Verification items for the finished model (mm, model axes). A direction names the side the tool comes from. Round coordinates to 2 decimals unless told otherwise and drop trailing zeros. Order: outer loops, then holes, each group sorted by start corner. A loop starts at its lowest first (then second) coordinate and runs counter-clockwise, first axis right, second up. Notation, with made-up numbers: (35, 64.5) -> (52, 64.5) arc R18 ccw to (52, 74.5) -> close; hole circle Ø10 at (9, 72.25). An arc over 180 degrees is marked (long way). Put each result on its own line as item: value.
Autodesk Inventor part; units mm, degrees
ref_plane "Work Plane1" through (29, 0, 0) normal (0, -1, 0) x (1, 0, 0)
ref_plane "YZ Plane" through (0, 0, 0) normal (1, 0, 0) x (0, 1, 0)
ref_plane "XZ Plane" through (0, 0, 0) normal (0, 1, 0) x (-1, 0, 0)
sketch "Sketch1" plane through (0, 0, 0) normal (0, 0, 1) x (1, 0, 0)
  line L0 (0.4667, 0) -> (20, 0)
  line L1 (20, 0) -> (20, 4)
  line L2 (20, 4) -> (1, 4)
  line L3 (1, 4) -> (0.2331, 4)
  line L4 (0.2331, 4) -> (0, 4)
  line L5 (0, 4) -> (0, 6.5)
  line L6 (0, 6.5) -> (-5, 6.5)
  line L7 (-5, 6.5) -> (-5, 2.8868)
  line L8 (-5, 2.8868) -> (-1.2, 2.8868)
  line L9 (-1.2, 2.8868) -> (0.4667, 0)
  line L10 (-7.5, 0) -> (27.5, 0)
  line L11 (0, -0.65) -> (0, 8.45)
  line L12 (1, 4) -> (0, 4) construction
  dimension "d1" = 19
  dimension "d2" = 0.7669
  dimension "d3" = 5
  dimension "d4" = 3.8
  dimension "d5" = 60
  dimension "d6" = 8
  dimension "d7" = 8
  dimension "d8" = 5.7735
  dimension "d9" = 13
  dimension "d26" = 20
revolve "Body" add sketch "Sketch1" angle 360 about axis through (0.4667, 0, 0) along (1, 0, 0) contours L9 L11 L4 L3 L2 L1 L0 | L9 L8 L7 L6 L5 L11
sketch "Sketch2" plane through (-5, 0, 0) normal (-1, 0, 0) x (0, 0, 1)
  circle A0 centre (0, 0) radius 2.8868
  line L0 (0, -7.8) -> (0, 10.4)
  line L1 (-7.8, 0) -> (10.4, 0)
  line L2 (2.8868, 0) -> (1.4434, -2.5)
  line L3 (1.4434, -2.5) -> (-1.4434, -2.5)
  line L4 (-1.4434, -2.5) -> (-2.8868, 0)
  line L5 (-2.8868, 0) -> (-1.4434, 2.5)
  line L6 (-1.4434, 2.5) -> (1.4434, 2.5)
  line L7 (1.4434, 2.5) -> (2.8868, 0)
  point P0 (0, 0)
extrude "Slot" add sketch "Sketch2" against normal up to next contours L7 A0 | A0 L2 | L6 L0 A0 | A0 L0 L3 | L0 L6 A0 | A0 L3 L0 | L4 A0 | A0 L5
fillet "Fillet1" radius 0.8 1 edges at (-5, -6.5, 0)
thread "Thread"
chamfer "Chamfer1" distance 0.7668 distance2 0.7668 1 edges at (20, -4, 0) measured on face at (20, -0.0467, 2.2623)
ref_plane "Work Plane1" through (29, 0, 0) normal (0, -1, 0) x (1, 0, 0)
equation "\"d17\" = RR"
equation "\"d15\" = -0.5 * SPD + 0.5 * GD"
equation "\"d16\" = GUL"
equation "\"d1\" = GEL"
equation "\"d3\" = KOH"
equation "\"d4\" = INTI"
equation "\"d6\" = GD"
equation "\"d7\" = BDM"
equation "\"d8\" = 1.1547 * SW"
equation "\"d9\" = KOD"
equation "\"d26\" = NLG"
equation "\"GD\" = NND"
equation "\"NLG\" = 20"
equation "\"GEL\" = 19"
equation "\"KOD\" = 13"
equation "\"KOH\" = 5"
equation "\"INTI\" = 3.8"
equation "\"GAL\" = 0.61345 * PTC"
equation "\"GUL\" = 0.61345 * PTC"
equation "\"BDM\" = NND"
equation "\"SW\" = 5"
equation "\"RR\" = 0.8"
equation "\"SPD\" = NND - 1.2269 * PTC"
equation "\"TOA\" = 30deg"
equation "\"GD1\" = THREADDIA - 1.2269 * PTC"
equation "\"THREADDIA\" = 8"
equation "\"FAWI\" = 45deg"
equation "\"ANG\" = 120deg"
equation "\"PTC\" = 1.25"
equation "\"NND\" = 8"
equation "\"E0\" = 1.155 * SW"
properties part number "21.1202" material "Steel, Mild"
Item 1: Release check for a two-part mould opening along Y. For faces 1 (the face through (20, 0, 0)), 2 (the face through (9.482, -0.867, 3.905)), 3 (the face through (-3, 2.5, 0)) record: pulls with the +Y half, pulls with the -Y half, needs draft (parallel to the pull), parting line crosses it, or undercut.
Geometry check:
face 1: needs draft
face 2: parting line crosses it
face 3: undercut
Item 2: Sectioned sample at A-A, the plane x = 3.5. Record the boundary of the cut face in (y, z).
Geometry check:
outline: circle Ø8 at (0, 0)
Item 3: Tool access check on faces 4 (the face through (0, 3, 3)), 5 (the face through (-3.017, 1.268, 2.155)), 6 (the face through (-2.129, -5.158, 3.955)). Record the directions out of +Z, -Z, +X, -X, +Y, -Y that give a thin tool (end or side, any length) a straight path to the whole face; none if there is none.
Geometry check:
face 4: +X
face 5: -X
face 6: +X, -X
Item 4: Material ranges on line 1 along X through (y, z) = (4.75, 2); line 2 along X through (y, z) = (-4.25, 4.75); line 3 along Z through (x, y) = (3.25, 3.25), recorded low to high.
Geometry check:
line 1: -5 to 0
line 2: -4.63 to 0
line 3: -2.33 to 2.33
Item 5: Depth check by flat-ended pin: pin 1 Ø6 at (x, y) = (14.5, 5) entering from +Z; pin 2 Ø6 at (x, z) = (0, -4.5) entering from +Y; pin 3 Ø1 at (x, z) = (12.5, 3.5) entering from +Y. Enter the tip coordinate at first touch or a pass-through.
Geometry check:
pin 1: z = 3.46
pin 2: y = 6.32
pin 3: y = 2.65
